The listing builds one solid part. Answer for the finished solid, in the listing's coordinates (mm). A direction names the side the tool comes from. Give positions to 0.01 mm unless a question says otherwise; leave off trailing zeros. Loops run counter-clockwise (first coordinate to the right, second up) from the corner with the lowest first, then second, coordinate; pieces in that order, holes last.
Item 1: Consider line 1 along Z through (x, y) = (1.5, 0.5); line 2 along X through (y, z) = (-1.25, -2.75); line 3 along X through (y, z) = (0.75, 0). Determine where each line is inside the solid, lowest interval first.
Item 2: This flat-tipped pin is pushed along its axis until it touches: pin 1 Ø2 at (x, y) = (3.5, -1) entering from +Z. Where does it stop, or does it pass through?
Item 3: The mould has two halves that part along Y. Classify faces 1 (the face through (12, 0, 0)), 2 (the face through (2.28, 0.09, -0.03)), 3 (the face through (2.37, -0.46, 2.06)): pulls with the +Y half, pulls with the -Y half, needs draft (parallel to the pull), parting line crosses it, or undercut.
Item 4: A tool of negligible diameter and unlimited length cuts with its end or side. For faces 4 (the face through (0.79, -0.63, -1.08)), 5 (the face through (0.363, -0.49, 3.733)), 6 (the face through (7, 0, 2)), from which of +Z, -Z, +X, -X, +Y, -Y can it reach the whole face along a straight path? Write none if from no direction.
Item 5: Section A-A, the plane x = 10.75 is taken. Give the vertices of the cut face in (y, z), and give its area (3 significant figures).
Autodesk Inventor part; units mm, degrees
ref_plane "Work Plane1" through (104.775, 0, 0) normal (0, 0, -1) x (1, 0, 0)
ref_plane "YZ Plane" through (0, 0, 0) normal (1, 0, 0) x (0, 1, 0)
ref_plane "XZ Plane" through (0, 0, 0) normal (0, 1, 0) x (-1, 0, 0)
sketch "Skizze1" plane through (0, 0, 0) normal (0, 0, 1) x (1, 0, 0)
  line L0 (12, 0) -> (12, 2)
  line L1 (12, 2) -> (4.58, 2)
  line L2 (4.58, 2) -> (4.1506, 2)
  line L3 (0, 3.765) -> (0, 1.4434)
  line L4 (0, 1.4434) -> (1.5, 1.4434)
  line L5 (1.5, 1.4434) -> (2.3333, 0)
  line L6 (2.3333, 0) -> (12, 0)
  line L7 (0, 3.765) -> (0.715, 3.765)
  line L8 (0.715, 3.765) -> (2.48, 2)
  line L9 (4.1506, 2) -> (2.48, 2)
  line L10 (4.58, 2) -> (2.48, 2) construction
  line L11 (2.48, 2) -> (2.48, 2)
  line L12 (-2.4, 0) -> (14.4, 0)
  line L13 (0, -0.753) -> (0, 4.518)
  dimension "d0" = 12
  dimension "d1" = 7.42
  dimension "d2" = 1.5
  dimension "d3" = 4
  dimension "d6" = 2.48
  dimension "d7" = 45
  dimension "d8" = 2.8868
  dimension "d9" = 60
  dimension "d10" = 7.53
  dimension "d11" = 4
  dimension "d12" = 0.4294
revolve "Körper" add sketch "Skizze1" angle 360 about axis through (2.3333, 0, 0) along (1, 0, 0) contours L6 L5 L4 L3 L7 L8 L9 L2 L1 L0
sketch "Skizze2" plane through (0, 0, 0) normal (-1, 0, 0) x (0, 0, 1)
  circle A0 centre (0, 0) radius 1.4434
  line L0 (0, -5.271) -> (0, 5.271)
  line L1 (-5.271, 0) -> (5.271, 0)
  line L2 (1.4434, 0) -> (0.7217, -1.25)
  line L3 (0.7217, -1.25) -> (-0.7217, -1.25)
  line L4 (-0.7217, -1.25) -> (-1.4434, 0)
  line L5 (-1.4434, 0) -> (-0.7217, 1.25)
  line L6 (-0.7217, 1.25) -> (0.7217, 1.25)
  line L7 (0.7217, 1.25) -> (1.4434, 0)
  point P0 (0, 1.4434)
extrude "Loch" add sketch "Skizze2" against normal up to next contours L7 A0 | A0 L2 | L6 L0 A0 | A0 L0 L3 | L0 L6 A0 | A0 L3 L0 | L4 A0 | A0 L5
thread "Gewinde"
chamfer "Fase1" distance 0.4294 distance2 0.4294 1 edges at (12, -2, 0) measured on face at (12, 0.3787, 0.698)
ref_plane "Work Plane1" through (104.775, 0, 0) normal (0, 0, -1) x (1, 0, 0)
equation "\"d15\" = GEL"
equation "\"d17\" = -0.5 * SPD + 0.5 * GD"
equation "\"d18\" = GUL"
equation "\"d0\" = NLG"
equation "\"d1\" = GEL"
equation "\"d2\" = INTI"
equation "\"d3\" = GD"
equation "\"d6\" = KOH"
equation "\"d7\" = 0.5 * SEWI"
equation "\"d8\" = 1.1547 * SW"
equation "\"d10\" = KOD"
equation "\"d11\" = BDM"
equation "\"d12\" = GAL"
equation "\"NLG\" = 12"
equation "\"INTI\" = 1.5"
equation "\"GEL\" = 7.42"
equation "\"GAL\" = 0.61345 * PTC"
equation "\"KOH\" = 2.48"
equation "\"KOD\" = 7.53"
equation "\"GUL\" = 0.61345 * PTC"
equation "\"SPD\" = NND - 1.2269 * PTC"
equation "\"BDM\" = NND"
equation "\"GD\" = NND"
equation "\"SEWI\" = 90deg"
equation "\"SW\" = 2.5"
equation "\"TOA\" = 30deg"
equation "\"GD1\" = THREADDIA - 1.2269 * PTC"
equation "\"EPV\" = 4.58"
equation "\"THREADDIA\" = 4"
equation "\"PTC\" = 0.7"
equation "\"NND\" = 4"
equation "\"E0\" = 2.89"
properties part number "ISO 10642  - M4  x  12" material "Stahl"
Worked answers:
1. line 1: z = -2.94 to -1.15, 1.15 to 2.94
1. line 2: x = 0 to 1.46
1. line 3: x = 1.9 to 12
2. pin 1: stops at z = 2
3. face 1: needs draft
3. face 2: undercut
3. face 3: parting line crosses it
4. face 4: -X
4. face 5: +X, -X
4. face 6: +X
5. outline: circle Ø4 at (0, 0)
5. area: 12.6 mm2
